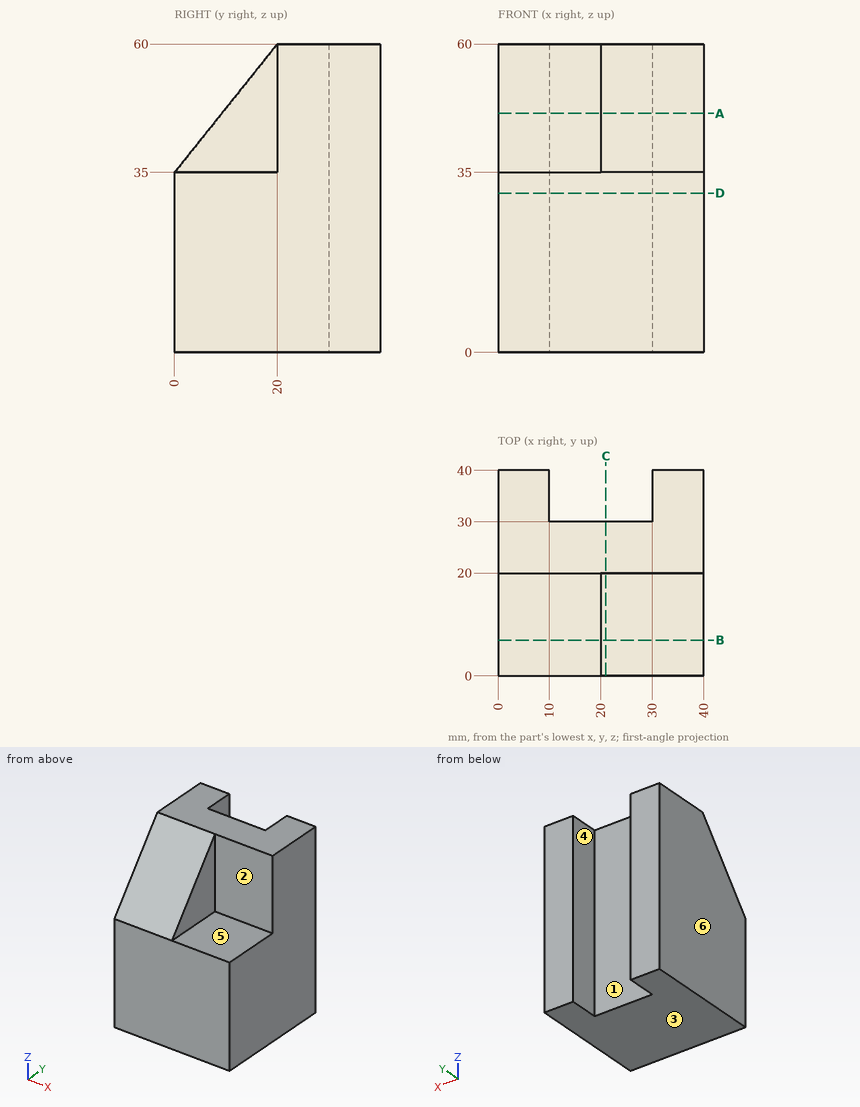
Print and shaded views of the part. All mm, measured from the part's lowest x, y and z. A direction names the side the tool comes from. Round coordinates to 2 decimals unless told otherwise and drop trailing zeros. Write each loop counter-clockwise with the first axis right and the second up, starting at its lowest first coordinate (ties: lowest second). Pieces come first, ordered by that corner, then holes. Notation, with made-up numbers: (1, -36.5) - (39, -36.5) arc R6 ccw to (39, -30.5) - close; hole circle Ø4 at (9, 44.5). An arc over 180 degrees is marked (long way). One line per question, with ' | ' between items.
1. Band-saw the part on C-C, the plane x = 21. Write the cut outline in (y, z).
Results are:
outline: (0, 0) - (30, 0) - (30, 60) - (20, 60) - (20, 35) - (0, 35) - close
2. Drop flat-ended pins along their axis: pin 1 Ø22 at (x, z) = (34, 48) entering from -Y; pin 2 Ø10 at (y, z) = (13.5, 42.5) entering from +X; pin 3 Ø3 at (x, z) = (19, 52.5) entering from -Y. Give the stop position or say it passes through.
Results are:
pin 1: y = 20 | pin 2: x = 20 | pin 3: y = 12.8
3. Mould opens along X. For the marked faces 4, 5 and 6 say: released by +X, released by -X, zero draft, split by the parting line, or undercut.
Results are:
face 4: undercut | face 5: zero draft | face 6: released by -X
4. Band-saw the part on D-D, the plane z = 31. Write the cut outline in (x, y).
Results are:
outline: (0, 0) - (40, 0) - (40, 40) - (30, 40) - (30, 30) - (10, 30) - (10, 40) - (0, 40) - close
5. Band-saw the part on B-B, the plane y = 7. Write the cut outline in (x, z), and give its area (4 significant figures).
Results are:
outline: (0, 0) - (40, 0) - (40, 35) - (20, 35) - (20, 43.75) - (0, 43.75) - close | area: 1,575 mm^2
6. Band-saw the part on A-A, the plane z = 46.5. Write the cut outline in (x, y).
Results are:
outline: (0, 9.2) - (20, 9.2) - (20, 20) - (40, 20) - (40, 40) - (30, 40) - (30, 30) - (10, 30) - (10, 40) - (0, 40) - close
7. Drill centre lines: line 1 along X through (y, z) = (36, 49.5); line 2 along Y through (x, z) = (21.5, 4); line 3 along Y through (x, z) = (35, 41). Where is each one in solid material? Low to high. Write a range as from..to.
Results are:
line 1: 0..10, 30..40 | line 2: 0..30 | line 3: 20..40
8. Tool access for the marked faces 1, 2 and 3: list every direction of +Z, -Z, +X, -X, +Y, -Y with a clear straight run to the whole face (end or side of a thin tool).
Results are:
face 1: +Z, -Z, +Y | face 2: +Z, +X, -Y | face 3: -Z, +X, -X, +Y, -Y
